Here's how the part is built. I have some questions about the finished solid (model axes, mm). Give positions to 0.01 mm unless a question says otherwise; leave off trailing zeros. Loops run counter-clockwise (first coordinate to the right, second up) from the corner with the lowest first, then second, coordinate; pieces in that order, holes last.
Q1. If we section it at B-B (y = 0): Please give me the cut outline in (x, z).
Q2. If we section it at C-C (z = -1.7): Please give me the cut outline in (x, y), plus the area to 3 significant figures.
Q3. If we section it at D-D (y = -14.5): Please give me the cut outline in (x, z), plus the area to 3 significant figures.
Q4. Will these pins go through, and if not, where does the flat tip stop? P1, Ø0.9, axis at x = -23.5, z = -2, coming from the -Y side; P2, Ø0.9, axis at y = -24, z = -1, coming from the -X side; P3, Ø0.9, axis at x = 18, z = -1.5, coming from the -Y side.
Q5. I need wall thicknesses on line 1 (Y direction, x = -0.1, z = -1.8); line 2 (X direction, y = 0, z = -1.65); line 3 (Y direction, x = 1.5, z = -1.2). Which ranges of each line are inside material? Lowest first, please.
Q6. If we section it at A-A (x = -0.1): Please give me the cut outline in (y, z).
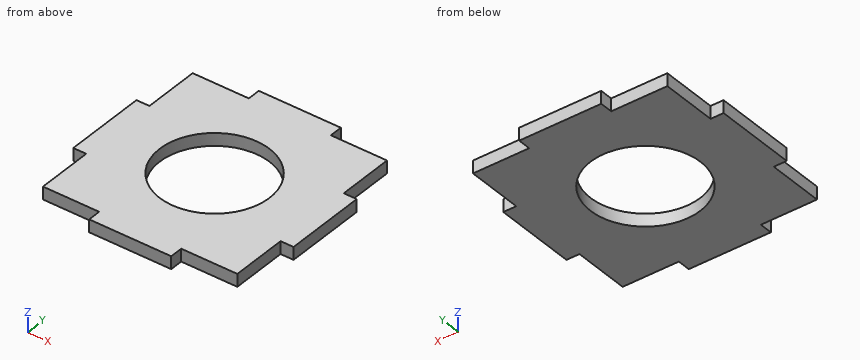
Autodesk Inventor part; units mm, degrees
ref_plane "XY Plane" through (0, 0, 0) normal (0, 0, 1) x (1, 0, 0)
sketch "Sketch1" plane through (0, 0, 0) normal (0, 0, 1) x (1, 0, 0)
  line L0 (-25.5, -25.5) -> (25.5, -25.5)
  line L1 (25.5, -25.5) -> (25.5, 25.5)
  line L2 (25.5, 25.5) -> (-25.5, 25.5)
  line L3 (-25.5, 25.5) -> (-25.5, -25.5)
  line L4 (-25.5, -25.5) -> (25.5, 25.5) construction
  line L5 (25.5, -25.5) -> (-25.5, 25.5) construction
  point P0 (0, 0)
  dimension "d0" = 51
  dimension "d1" = 51
extrude "Extrusion1" add sketch "Sketch1" against normal blind 2.921
sketch "Sketch2" plane through (0, 0, 0) normal (0, 0, 1) x (1, 0, 0)
  line L0 (-25.5, 25.5) -> (-9.5, 25.5)
  line L1 (-9.5, 25.5) -> (-9.5, 22.5)
  line L2 (-9.5, 22.5) -> (-22.5, 22.5)
  line L3 (-25.5, 22.4108) -> (-25.5, 25.5)
  line L4 (-25.5, 25.5) -> (-22.225, 25.5)
  line L5 (-22.5, 22.5) -> (-22.5, 9.5)
  line L6 (-22.5, 9.5) -> (-25.5, 9.5)
  line L7 (-25.5, 9.5) -> (-25.5, 25.5)
  line L8 (25.5, 25.5) -> (-25.5, 25.5)
  line L9 (-25.5, 25.5) -> (-25.5, -25.5)
  dimension "d59" = 3
  dimension "d62" = 3
  dimension "d67" = 16
  dimension "d73" = 16
hole "Hole1" at (-0.1, 0, 0) direction (0, 0, -1) diameter 25.4 end through all
extrude "Extrusion4" cut sketch "Sketch2" against normal up to next
mirror "Mirror1" about plane through (0, 0, 0) normal (1, 0, 0) of "Extrusion4"
mirror "Mirror2" about plane through (0, 0, 0) normal (0, 1, 0) of "Extrusion4", "Mirror1"
equation "\"d1\" = d0"
equation "\"d62\" = d59"
equation "\"d67\" = d73"
equation "\"d53\" = 0.5 * d0"
properties part number "Top"
Check sheet entries:
1. outline: (-25.5, -2.92) - (-12.8, -2.92) - (-12.8, 0) - (-25.5, 0) - close; (12.6, -2.92) - (25.5, -2.92) - (25.5, 0) - (12.6, 0) - close
2. outline: (-25.5, -9.5) - (-22.5, -9.5) - (-22.5, -22.5) - (-9.5, -22.5) - (-9.5, -25.5) - (9.5, -25.5) - (9.5, -22.5) - (22.5, -22.5) - (22.5, -9.5) - (25.5, -9.5) - (25.5, 9.5) - (22.5, 9.5) - (22.5, 22.5) - (9.5, 22.5) - (9.5, 25.5) - (-9.5, 25.5) - (-9.5, 22.5) - (-22.5, 22.5) - (-22.5, 9.5) - (-25.5, 9.5) - close; hole circle Ø25.4 at (-0.1, 0)
2. area: 1,750 mm2
3. outline: (-22.5, -2.92) - (22.5, -2.92) - (22.5, 0) - (-22.5, 0) - close
3. area: 131 mm2
4. P1: stops at y = -9.5
4. P2: stops at x = -9.5
4. P3: stops at y = -22.5
5. line 1: y = -25.5 to -12.7, 12.7 to 25.5
5. line 2: x = -25.5 to -12.8, 12.6 to 25.5
5. line 3: y = -25.5 to -12.6, 12.6 to 25.5
6. outline: (-25.5, -2.92) - (-12.7, -2.92) - (-12.7, 0) - (-25.5, 0) - close; (12.7, -2.92) - (25.5, -2.92) - (25.5, 0) - (12.7, 0) - close
